Build history of the part. All positions in model axes, mm. Face numbers are marked on the shaded views. Round coordinates to 2 decimals unless told otherwise and drop trailing zeros. Write each loop counter-clockwise with the first axis right and the second up, starting at its lowest first coordinate (ties: lowest second). Pieces come first, ordered by that corner, then holes. Notation, with made-up numbers: (68, 10.5) - (90, 10.5) arc R19 cw to (90, 43.5) - close; hole circle Ø3 at (-38.75, 19.5). An arc over 180 degrees is marked (long way). Write each question's results on one line, items separated by ' | '.
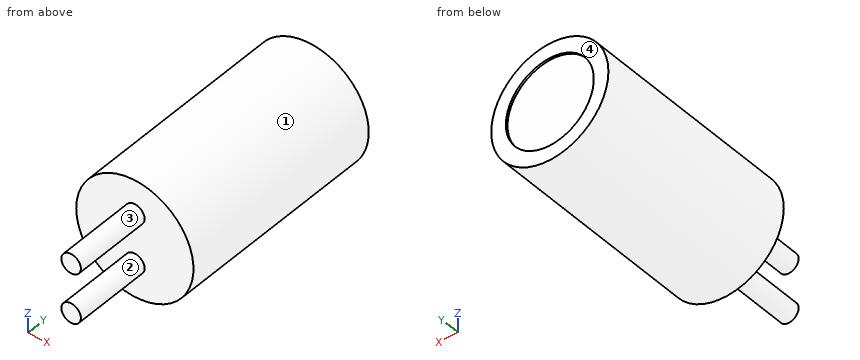
Autodesk Inventor part; units mm, degrees
ref_plane "Arbeitsebene1" through (-1.5, 0, 0) normal (1, 0, 0) x (0, 1, 0)
ref_plane "Arbeitsebene2" through (1.5, 0, 0) normal (1, 0, 0) x (0, 1, 0)
ref_plane "Arbeitsebene3" through (-0.5, 0, 0) normal (1, 0, 0) x (0, 1, 0)
sketch "Skizze3" plane through (0, 0, 0) normal (0, 1, 0) x (-1, 0, 0)
  circle A0 centre (0, 0) radius 3
  dimension "Durchmesser" = 6
extrude "Extrusion2" add sketch "Skizze3" along normal blind 11
sketch "Skizze4" plane through (0, 0, 0) normal (0, -1, 0) x (1, 0, 0)
  circle A0 centre (0, 1.27) radius 0.5
  circle A1 centre (0, -1.27) radius 0.5
  point P0 (0, 0)
  dimension "d6" = 1
  dimension "d7" = 1
  dimension "BeinAbstand" = 2.54
  dimension "BeinZuMitte" = 1.27
extrude "Extrusion3" add sketch "Skizze4" along normal blind 4
ref_plane "Arbeitsebene1" through (-1.5, 0, 0) normal (1, 0, 0) x (0, 1, 0)
ref_plane "Arbeitsebene2" through (1.5, 0, 0) normal (1, 0, 0) x (0, 1, 0)
split_face "Trennen1"
split_face "Trennen2"
ref_plane "Arbeitsebene3" through (-0.5, 0, 0) normal (1, 0, 0) x (0, 1, 0)
ref_plane "Arbeitsebene4" through (0.5, 0, 0) normal (1, 0, 0) x (0, 1, 0)
ref_plane "Arbeitsebene5" through (0, 9, 0) normal (0, 1, 0) x (1, 0, 0)
ref_plane "Arbeitsebene6" through (0, 6.5, 0) normal (0, 1, 0) x (1, 0, 0)
sketch "Skizze5" plane through (0, 11, 0) normal (0, 1, 0) x (1, 0, 0)
  circle A0 centre (0, 0) radius 2.25
  dimension "d21" = 4.5
extrude "Extrusion4" cut sketch "Skizze5" against normal blind 0.1
split_face "Trennen3"
split_face "Trennen4"
split_face "Trennen7"
split_face "Trennen8"
ref_plane "Arbeitsebene9" through (0, 3.5, 0) normal (0, -1, 0) x (1, 0, 0)
ref_plane "Arbeitsebene10" through (0, 1, 0) normal (0, -1, 0) x (1, 0, 0)
split_face "Trennen9"
split_face "Trennen10"
properties part number "Kondensator"
(1) Slice it at D-D, the plane x = -1.2. Write the cut outline in (y, z).
Worked answers:
outline: (0, -2.75) - (11, -2.75) - (11, -1.9) - (10.9, -1.9) - (10.9, 1.9) - (11, 1.9) - (11, 2.75) - (0, 2.75) - close
(2) Flat gauge pins, fed straight in: pin 1 Ø1.5 at (y, z) = (3, -2.5) entering from +X; pin 2 Ø1.3 at (x, z) = (0, 1) entering from +Y; pin 3 Ø1 at (x, y) = (-1, 5) entering from -Z. Where does each tip first touch, or does it go through?
Worked answers:
pin 1: stops at x = 2.44 | pin 2: stops at y = 10.9 | pin 3: stops at z = -2.96
(3) Slice it at A-A, the plane z = 0. Write the cut outline in (x, y).
Worked answers:
outline: (-3, 0) - (3, 0) - (3, 11) - (2.25, 11) - (2.25, 10.9) - (-2.25, 10.9) - (-2.25, 11) - (-3, 11) - close
(4) Two-plate mould, pull along Z, no slides. Class the marked faces 1, 2, 3 and 4: released by +Z, released by -Z, zero draft, split by the parting line, or undercut.
Worked answers:
face 1: split by the parting line | face 2: undercut | face 3: undercut | face 4: zero draft
(5) Slice it at B-B, the plane x = 0. Write the cut outline in (y, z).
Worked answers:
outline: (-4, -1.77) - (0, -1.77) - (0, -3) - (11, -3) - (11, -2.25) - (10.9, -2.25) - (10.9, 2.25) - (11, 2.25) - (11, 3) - (0, 3) - (0, 1.77) - (-4, 1.77) - (-4, 0.77) - (0, 0.77) - (0, -0.77) - (-4, -0.77) - close
(6) Drill centre lines: probe 1 along Z at (x, y) = (0, 10.95); probe 2 along Y at (x, z) = (2.55, 0.95); probe 3 along Y at (x, z) = (-1.2, 1.4). Where is each one in solid material? Low to high. Write a range as [from, to].
Worked answers:
probe 1: z = [-3, -2.25], [2.25, 3] | probe 2: y = [0, 11] | probe 3: y = [0, 10.9]
(7) Slice it at C-C, the plane y = 0.25. Write the cut outline in (x, z), and give its area (3 significant figures).
Worked answers:
outline: circle Ø6 at (0, 0) | area: 28.3 mm2
